Input: part model. Units: mm. Frame: model coordinates. A direction names the side the tool comes from. Coordinates: 2 decimals unless noted, no trailing zeros. Order: outer loops, then holes, each group sorted by start corner. A loop starts at its lowest first (then second) coordinate and runs counter-clockwise, first axis right, second up. Notation, with made-up numbers: (-14.5, -39.75) -> (1.5, -39.75) arc R20 ccw to (1.5, -12.75) -> close; hole circle Ø6 at (25, 73.25). An arc over 180 degrees is marked (long way). Use one line per item in the form item = value. Start each with the question number.
1) Ray query, line 1 along Y through (x, z) = (0, 3.5) (3 decimals); line 2 along X through (y, z) = (30.5, 6) (3 decimals); line 3 along Y through (x, z) = (19, 6.5). Return the intervals inside material, ascending.
2) Access query for faces 4 (the flat face through (0, 30.338, 5)), 5 (the flat face through (-14.216, -29.776, 5.116)), 6 (the flat face through (-8.27, -32.01, 5.12)). Directions: +Z, -Z, +X, -X, +Y, -Y. A direction counts if a zero-diameter tool reaches every point of the face in a straight line with its end or side. Return the directions, or none.
3) Section query A-A on y = 0. Output: boundary loops of the cut face in (x, z) (3 decimals), then the cut area to 3 significant figures.
4) Pin query (flat end, axial travel): pin 1 (2 mm diameter, centred on x = -12.5, y = -29.5, fed in from +Z); pin 2 (5.5 mm diameter, centred on x = 1, y = -33.5, fed in from +Z); pin 3 (1.5 mm diameter, centred on y = 32.5, z = 4, fed in from -X); pin 4 (1 mm diameter, centred on y = 18.5, z = 4, fed in from -X). Return the tip coordinate at first contact, or that it passes through.
5) Section query D-D on x = 18.5. Output: boundary loops of the cut face in (y, z), then the cut area to 3 significant figures.
6) Section query C-C on z = 1. Output: boundary loops of the cut face in (x, y) (3 decimals), then the cut area to 3 significant figures.
7) Section query B-B on x = 0. Output: boundary loops of the cut face in (y, z) (3 decimals).
8) Draft query along X for faces 1 (the flat face through (-18.72, -27.25, 5.12)), 2 (the flat face through (-21, -25, 2.54)), 3 (the flat face through (18.72, 27.25, 5.12)). Return one class per face: pulls with the +X half, pulls with the -X half, needs draft (parallel to the pull), parting line crosses it, or undercut.
from build123d import *

# Parameters (mm, degrees)
F0_R            = 35.56
F0_R_2          = 23.495
F1_DEPTH        = 7.62
F3_DEPTH        = 5.08
F3_COPIES_COUNT = 18


# Not quite as in the source:
# - a pattern or mirror of a feature is missing from the dataset's text; its kind, count and spacing are read off the source's solid


with BuildPart() as f1:
    # F0 (on Top) → F1 (new body)
    with BuildSketch(Plane.XY):
        Circle(F0_R)
        Circle(F0_R_2, mode=Mode.SUBTRACT)
    extrude(amount=F1_DEPTH)

    # F2 (on face) → F3 (cut)
    with BuildSketch(Plane.XY.offset(7.62)):
        with BuildLine():
            Line((-3.175, -30.3379753092), (-3.175, -35.4179753092))
            ThreePointArc((-3.175, -35.4179753092), (0, -35.56), (3.175, -35.4179753092))
            Line((3.175, -35.4179753092), (3.175, -30.3379753092))
            Line((3.175, -30.3379753092), (-3.175, -30.3379753092))
        make_face()
    f3 = extrude(amount=-F3_DEPTH, mode=Mode.SUBTRACT)

    # F3_copies: F3 ×18 about axis
    f3_copies_axis = Axis((0, 0, 0), (0, 0, 1))
    for i in range(1, F3_COPIES_COUNT):
        add(f3.rotate(f3_copies_axis, i * 360 / F3_COPIES_COUNT), mode=Mode.SUBTRACT)


solid = f1.part
Answers below:
q1.line_1 = -30.338 to -23.495, 23.495 to 30.338
q1.line_2 = -18.283 to -14.48, -7.722 to -3.175, 3.175 to 7.722, 14.48 to 18.283
q1.line_3 = -30.06 to -27.58, -23.66 to -13.82, 13.82 to 23.66, 27.58 to 30.06
q2.face_4 = +Z, +Y
q2.face_5 = +Z, -Y
q2.face_6 = +Z
q3.outline = (-35.56, 0) -> (-23.495, 0) -> (-23.495, 7.62) -> (-35.56, 7.62) -> close; (23.495, 0) -> (35.56, 0) -> (35.56, 7.62) -> (23.495, 7.62) -> close
q3.area = 184 mm^2
q4.pin_1 = 2.54
q4.pin_2 = 7.62
q4.pin_3 = -16.01
q4.pin_4 = -26.56
q5.outline = (-30.37, 0) -> (-14.48, 0) -> (-14.48, 7.62) -> (-24.08, 7.62) -> (-24.08, 2.54) -> (-26.99, 2.54) -> (-26.99, 7.62) -> (-30.37, 7.62) -> close; (14.48, 0) -> (30.37, 0) -> (30.37, 7.62) -> (26.99, 7.62) -> (26.99, 2.54) -> (24.08, 2.54) -> (24.08, 7.62) -> (14.48, 7.62) -> close
q5.area = 213 mm^2
q6.outline = circle Ø71.12 at (0, 0); hole circle Ø46.99 at (0, 0)
q6.area = 2,240 mm^2
q7.outline = (-35.56, 0) -> (-23.495, 0) -> (-23.495, 7.62) -> (-30.338, 7.62) -> (-30.338, 2.54) -> (-35.56, 2.54) -> close; (23.495, 0) -> (35.56, 0) -> (35.56, 2.54) -> (30.338, 2.54) -> (30.338, 7.62) -> (23.495, 7.62) -> close
q8.face_1 = pulls with the -X half
q8.face_2 = undercut
q8.face_3 = pulls with the +X half
